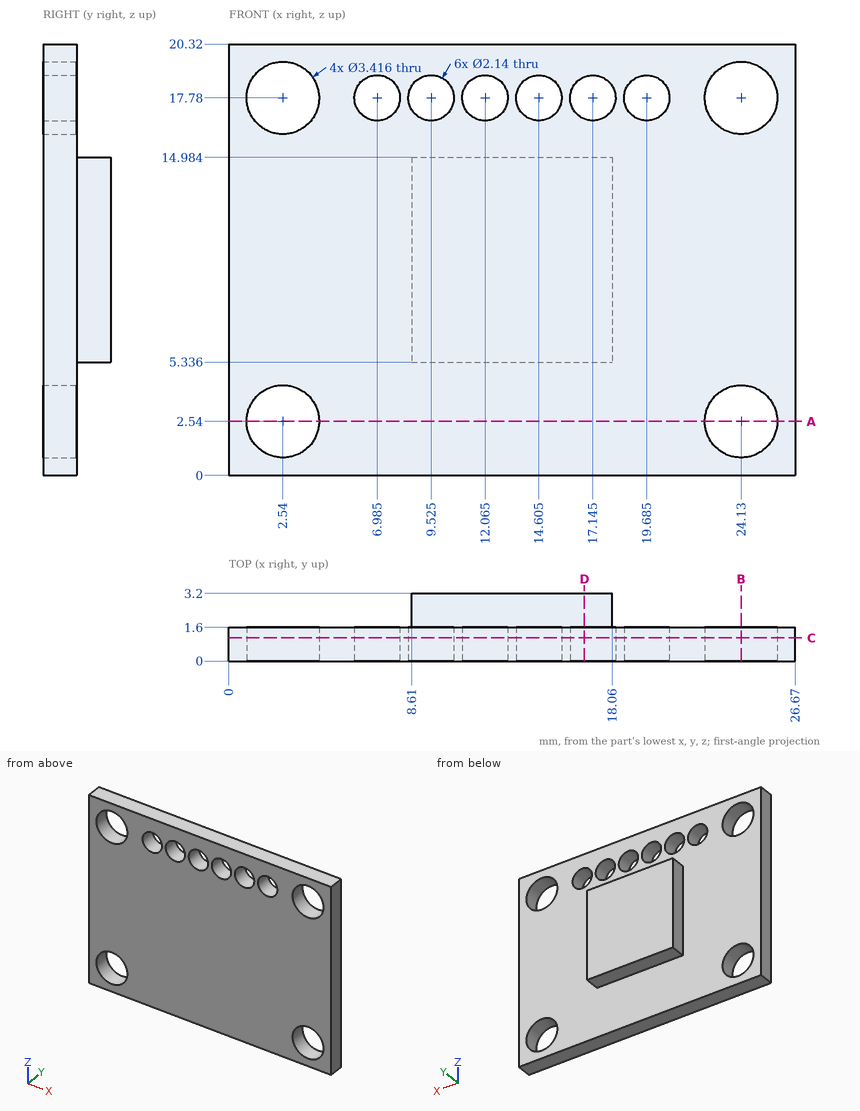
Print and shaded views of the part. All mm, measured from the part's lowest x, y and z. Give positions to 0.01 mm unless a question says otherwise; leave off trailing zeros. Loops run counter-clockwise (first coordinate to the right, second up) from the corner with the lowest first, then second, coordinate; pieces in that order, holes last. Notation, with made-up numbers: (-25.75, -7.75) - (9.25, -7.75) arc R23 cw to (9.25, 31.25) - close; hole circle Ø5 at (18.25, -10.75). An arc over 180 degrees is marked (long way). One line per item, written item: value. Start each with the question number.
1. Probe L1, parallel to X at y = 0.6, z = 2.54; L2, parallel to Z at x = 2.75, y = 0.4 (1 decimal); L3, parallel to Z at x = 14.5, y = 1.2 (1 decimal). List the from-to ranges inside material, lowest first. Write a range as from..to.
2. Slice it at A-A (z = 2.54). List the corners of the cut face in (x, y).
3. Slice it at B-B (x = 24.13). List the corners of the cut face in (y, z).
4. Slice it at C-C (y = 1.1). Give the number of separate pieces and of enclosed holes in the cut face, plus the area to 3 significant figures.
5. Slice it at D-D (x = 16.75). List the corners of the cut face in (y, z) (1 decimal).
6. Pin check, flat tips, straight feed: pin 1 (1.9 mm diameter, centred on x = 17.145, z = 17.78, fed in from +Y); pin 2 (3 mm diameter, centred on x = 12.065, z = 17.78, fed in from +Y); pin 3 (1.3 mm diameter, centred on x = 13, y = 2.5, fed in from -Z). Stop position of each tip, or through.
Solution:
1. L1: x = 0..0.83, 4.25..22.42, 25.84..26.67
1. L2: z = 0..0.8, 4.2..16.1, 19.5..20.3
1. L3: z = 0..16.7, 18.8..20.3
2. outline: (0, 0) - (0.83, 0) - (0.83, 1.6) - (0, 1.6) - close; (4.25, 0) - (22.42, 0) - (22.42, 1.6) - (4.25, 1.6) - close; (25.84, 0) - (26.67, 0) - (26.67, 1.6) - (25.84, 1.6) - close
3. outline: (0, 0) - (1.6, 0) - (1.6, 0.83) - (0, 0.83) - close; (0, 4.25) - (1.6, 4.25) - (1.6, 16.07) - (0, 16.07) - close; (0, 19.49) - (1.6, 19.49) - (1.6, 20.32) - (0, 20.32) - close
4. separate pieces: 1
4. enclosed holes: 10
4. area: 484 mm^2
5. outline: (0, 0) - (1.6, 0) - (1.6, 5.3) - (3.2, 5.3) - (3.2, 15) - (1.6, 15) - (1.6, 16.8) - (0, 16.8) - close; (0, 18.8) - (1.6, 18.8) - (1.6, 20.3) - (0, 20.3) - close
6. pin 1: passes through
6. pin 2: stops at y = 1.6
6. pin 3: stops at z = 5.34
